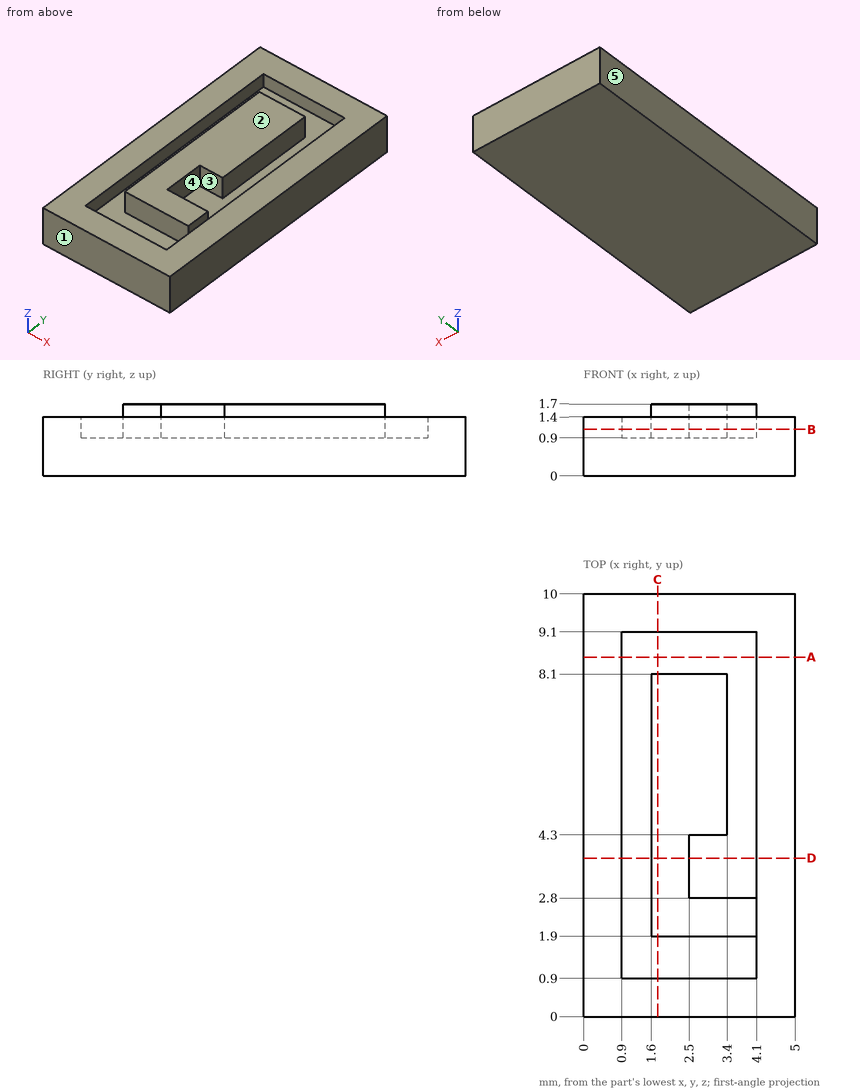
The drawing under review shows one solid part. Ordinate dimensions are in mm from its lowest x, y, z. A direction names the side the tool comes from. Coordinates: 2 decimals unless noted, no trailing zeros. Write each loop counter-clockwise with the first axis right and the second up, starting at its lowest first coordinate (ties: lowest second). Pieces come first, ordered by that corner, then holes.
1) Add section D-D (y = 3.75). Write out the cut boundary in (x, z), plus the area to 3 significant figures.
2) Add section C-C (x = 1.75). Write out the cut boundary in (y, z), plus the area to 3 significant figures.
3) Mouldability with a two-part tool opening along Y and no side actions: class the marked faces 1, 2 and 3 as +Y half, -Y half, draft (parallel to the pull), parting line (faces both ways), or undercut.
4) Add section B-B (z = 1.1). Write out the cut boundary in (x, y).
5) Machinability: for the marked faces 4 and 5, which of the approach directions +Z, -Z, +X, -X, +Y, -Y give a long, thin tool a straight path to every point of the face, cutting with its end or side? Answer none if there is none.
6) Add section A-A (y = 8.5). Write out the cut boundary in (x, z).
7) To check wall thickness, follow L1, parallel to X at y = 4.25, z = 1.3; L2, parallel to X at y = 6.25, z = 1; L3, parallel to Y at x = 4.05, z = 1.2. State the ranges of each line that lie inside material, in increasing order.
Check result:
1. outline: (0, 0) - (5, 0) - (5, 1.4) - (4.1, 1.4) - (4.1, 0.9) - (2.5, 0.9) - (2.5, 1.7) - (1.6, 1.7) - (1.6, 0.9) - (0.9, 0.9) - (0.9, 1.4) - (0, 1.4) - close
1. area: 6.12 mm2
2. outline: (0, 0) - (10, 0) - (10, 1.4) - (9.1, 1.4) - (9.1, 0.9) - (8.1, 0.9) - (8.1, 1.7) - (1.9, 1.7) - (1.9, 0.9) - (0.9, 0.9) - (0.9, 1.4) - (0, 1.4) - close
2. area: 14.9 mm2
3. face 1: -Y half
3. face 2: draft
3. face 3: undercut
4. outline: (0, 0) - (5, 0) - (5, 10) - (0, 10) - close; hole (0.9, 0.9) - (4.1, 0.9) - (4.1, 1.9) - (1.6, 1.9) - (1.6, 8.1) - (3.4, 8.1) - (3.4, 4.3) - (2.5, 4.3) - (2.5, 2.8) - (4.1, 2.8) - (4.1, 9.1) - (0.9, 9.1) - close
5. face 4: +Z
5. face 5: +Z, -Z, -X, +Y, -Y
6. outline: (0, 0) - (5, 0) - (5, 1.4) - (4.1, 1.4) - (4.1, 0.9) - (0.9, 0.9) - (0.9, 1.4) - (0, 1.4) - close
7. L1: x = 0 to 0.9, 1.6 to 2.5, 4.1 to 5
7. L2: x = 0 to 0.9, 1.6 to 3.4, 4.1 to 5
7. L3: y = 0 to 0.9, 1.9 to 2.8, 9.1 to 10
